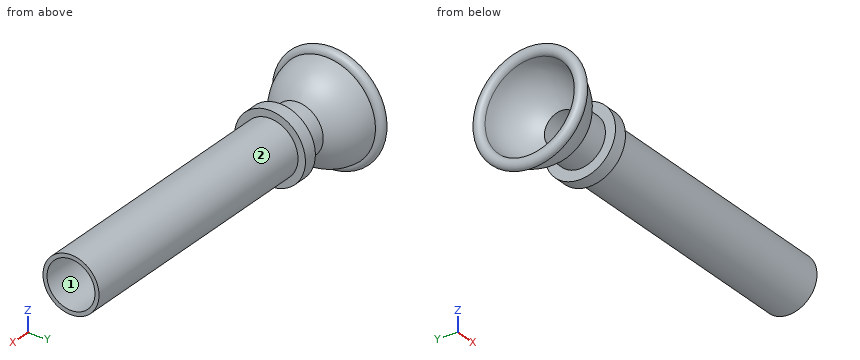
from build123d import *


with BuildPart() as part:
    # Sketch1 → Revolve1 (revolve)
    with BuildSketch(Plane.XY, mode=Mode.PRIVATE) as revolve1_sk:
        with BuildLine():
            Line((117.55898886, 6.49609803), (15.95898886, 6.49609803))
            Line((15.95898886, 6.49609803), (15.95898886, 3.82909803))
            Line((15.95898886, 3.82909803), (10.87898886, 3.82909803))
            Line((10.87898886, 3.82909803), (1.267903452, 3.82909803))
            ThreePointArc((1.267903452, 3.82909803), (-4.993471479, 11.580101966), (-14.52101114, 14.49709803))
            ThreePointArc((-14.52101114, 14.49709803), (-15.827069138, 18.085772853), (-12.519920979, 16.176022729))
            ThreePointArc((-12.519920979, 16.176022729), (-4.32104899, 13.27593718), (1.696011458, 6.996846349))
            Line((1.696011458, 6.996846349), (10.87898886, 6.996846349))
            Line((10.87898886, 6.996846349), (10.87898886, 10.81409803))
            Line((10.87898886, 10.81409803), (15.95898886, 10.81409803))
            Line((15.95898886, 10.81409803), (15.95898886, 8.02009803))
            Line((15.95898886, 8.02009803), (117.55898886, 8.02009803))
            Line((117.55898886, 8.02009803), (117.55898886, 6.49609803))
        make_face()
    revolve(revolve1_sk.sketch.rotate(Axis((-17.599665341, -2.52090197, 0), (1, 0, 0)), 90), axis=Axis((-17.599665341, -2.52090197, 0), (1, 0, 0)))


solid = part.part
For this review, take the finished solid that the model builds, in its own axes (mm). Face numbers are marked on the shaded views. Give positions to 0.01 mm unless a question says otherwise; leave off trailing zeros. Loops run counter-clockwise (first coordinate to the right, second up) from the corner with the lowest first, then second, coordinate; pieces in that order, holes last. Notation, with made-up numbers: M -36,45.25 L -15,45.25 A22 ccw -15,81.25 Z; hole C -30,46 d8. An arc over 180 degrees is marked long. Answer as a JSON object with one key per item and string values. Group by question number.
Q1. Add section B-B on x = 41. Give the boundary of the cut face in (y, z), and give its area (3 significant figures).
Q2. Mouldability with a two-part tool opening along Z and no side actions: class the marked faces 1 and 2 as +Z half, -Z half, draft (parallel to the pull), parting line (faces both ways), or undercut.
Q3. Insertion check: P1, Ø14.5, axis at y = -2.52, z = 0, coming from the -X side (3 decimals); P2, Ø21.5, axis at y = -2, z = -6.5, coming from the -X side; P3, Ø6, axis at x = 38, z = 12.5, coming from the -Y side. Each pin has a flat end and moves straight along its axis. Give the tip position at first contact, or say it passes through.
Q4. For probe 1 along Y at (x, z) = (70, 0); probe 2 along Y at (x, z) = (6.5, 0); probe 3 along Z at (x, y) = (3.5, -6.5), list the stretches that pass through material, from the lowest coordinate up. Write a range as [from, to].
Q5. Add section A-A on z = 0. Give the boundary of the cut face in (x, y), and give its area (3 significant figures).
Checked values:
{
 "1": {"outline": "C -2.52,0 d21.08; hole C -2.52,0 d18.03", "area": "93.6 mm²"},
 "2": {"face 1": "undercut", "face 2": "parting line"},
 "3": {"P1": "x = 0.875", "P2": "x = -15.5", "P3": "y = -7.09"},
 "4": {"probe 1": "[-13.06, -11.54], [6.5, 8.02]", "probe 2": "[-12.04, -8.87], [3.83, 7]", "probe 3": "[-8.65, -4.95], [4.95, 8.65]"},
 "5": {"outline": "M -14.52,-19.54 A2.03 ccw long -12.52,-21.22 A18.8 ccw 1.7,-12.04 L 10.88,-12.04 L 10.88,-15.86 L 15.96,-15.86 L 15.96,-13.06 L 117.56,-13.06 L 117.56,-11.54 L 15.96,-11.54 L 15.96,-8.87 L 1.27,-8.87 A17.02 cw Z; M -14.52,14.5 A17.02 cw 1.27,3.83 L 15.96,3.83 L 15.96,6.5 L 117.56,6.5 L 117.56,8.02 L 15.96,8.02 L 15.96,10.81 L 10.88,10.81 L 10.88,7 L 1.7,7 A18.8 ccw -12.52,16.18 A2.03 ccw long Z", "area": "532 mm²"}
}
